Autodesk Inventor part; units mm, degrees
ref_plane "YZ Plane" through (0, 0, 0) normal (1, 0, 0) x (0, 1, 0)
ref_plane "XZ Plane" through (0, 0, 0) normal (0, 1, 0) x (-1, 0, 0)
ref_plane "XY Plane" through (0, 0, 0) normal (0, 0, 1) x (1, 0, 0)
sketch "Sketch1" plane through (0, 0, 0) normal (0, 0, 1) x (1, 0, 0)
  line L0 (-17, 28) -> (0, 28)
  line L1 (0, 28) -> (0, 0)
  line L2 (0, 0) -> (-17, 0)
  line L3 (-17, 0) -> (-17, 28)
  dimension "d0" = 17
  dimension "d1" = 28
extrude "Extrusion1" add sketch "Sketch1" along normal blind 1
sketch "Sketch2" plane through (0, 0, 1) normal (0, 0, 1) x (1, 0, 0)
  line L0 (-17, 28) -> (-17, 0)
  line L1 (0, 28) -> (-17, 28)
  line L2 (0, 0) -> (0, 28)
  line L3 (-17, 0) -> (0, 0)
  circle A0 centre (-12.5, 26) radius 1.35
  circle A1 centre (-4.5, 5) radius 1.35
  dimension "d4" = 2.7
  dimension "d5" = 2.7
  dimension "d6" = 4.5
  dimension "d7" = 4.5
  dimension "d8" = 2
  dimension "d9" = 5
extrude "Extrusion2" cut sketch "Sketch2" against normal through all contours A0 | A1
sketch "Sketch3" plane through (0, 0, 1) normal (0, 0, 1) x (1, 0, 0)
  circle A0 centre (-12.5, 26) radius 1.35
  circle A1 centre (-4.5, 5) radius 1.35
  line L0 (0, 28) -> (-17, 28)
  line L1 (-17, 28) -> (-17, 0)
  line L2 (-17, 0) -> (0, 0)
  line L3 (0, 0) -> (0, 28)
  circle A2 centre (-8.5, 12.047) radius 6.5
  dimension "d12" = 13
  dimension "d13" = 12.047
extrude "Extrusion3" add sketch "Sketch3" along normal blind 30 contours A2
sketch "Sketch4" plane through (-8.5, 12.047, 31) normal (0, 0, 1) x (1, 0, 0)
  circle A0 centre (0, 0) radius 6.5
  circle A1 centre (0, 0) radius 3.25
  point P0 (8.5, -12.047)
  dimension "d16" = 6.5
sketch "Sketch5" plane through (0, 0, 0) normal (0, 0, -1) x (-1, 0, 0)
  circle A0 centre (8.5, 12.047) radius 6.5
  circle A1 centre (8.5, 12.047) radius 5
  point P0 (0, 0)
  dimension "d17" = 10
loft "Loft1" cut profiles "Sketch5", "Sketch4" contours A1 / A1
sketch "Sketch6" plane through (-8.5, 12.047, 31) normal (0, 0, 1) x (1, 0, 0)
  circle A0 centre (0, 0) radius 3.25
  circle A1 centre (0, 0) radius 4.75
  point P0 (8.5, -12.047)
  dimension "d26" = 9.5
extrude "Extrusion6" add sketch "Sketch6" along normal blind 3
sketch "Sketch7" plane through (-8.5, 12.047, 34) normal (0, 0, 1) x (1, 0, 0)
  circle A0 centre (0, 0) radius 3.25
  circle A1 centre (0, 0) radius 4.75
  line L0 (2, 0) -> (-2, 0)
  line L1 (-2, 0) -> (-2, 6)
  line L2 (-2, 6) -> (2, 6)
  line L3 (2, 6) -> (2, 0)
  point P0 (8.5, -12.047)
  dimension "d29" = 4
  dimension "d30" = 2
extrude "Extrusion7" cut sketch "Sketch7" against normal up to surface (3 mm away) contours L3 L0 L1 A0 | A0 L1 A1 L3 | A1 L1 L2 L3 picked at (0, 1.0833) picked at (0.3414, 4.2128)
properties part number "TORRE0.2"
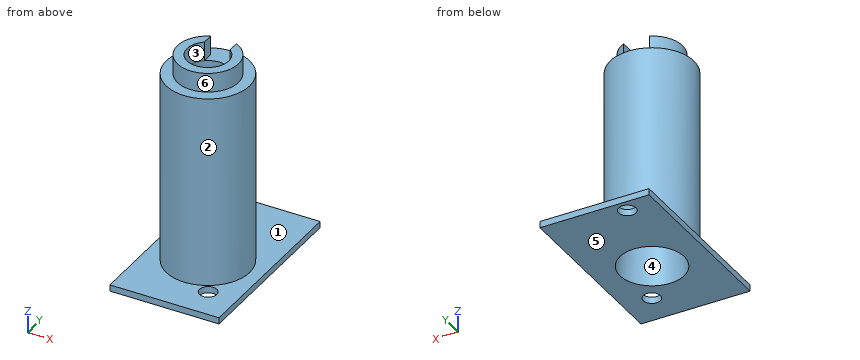
Build history of the part. All positions in model axes, mm. Face numbers are marked on the shaded views. A direction names the side the tool comes from. Give positions to 0.01 mm unless a question says otherwise; leave off trailing zeros. Write each loop counter-clockwise with the first axis right and the second up, starting at its lowest first coordinate (ties: lowest second). Pieces come first, ordered by that corner, then holes. Notation, with made-up numbers: (61.5, 40.25) - (72.5, 40.25) arc R21 ccw to (72.5, 60.25) - close; hole circle Ø8 at (86.25, 73.25). An arc over 180 degrees is marked (long way). Use one line per item in the form item = value. Start each with the question number.
1. Band-saw the part on B-B on x = -8.5. Write the cut outline in (y, z).
2. Band-saw the part on A-A on y = 26. Write the cut outline in (x, z).
3. Drop flat-ended pins along their axis: pin 1 Ø4 at (x, y) = (-5, 23.5) entering from +Z; pin 2 Ø6 at (y, z) = (12.5, 29.5) entering from +X; pin 3 Ø3 at (x, y) = (-10.5, 16) entering from -Z; pin 4 Ø3 at (x, y) = (-2.5, 7) entering from +Z. Give the stop position or say it passes through.
4. Band-saw the part on C-C on z = 12. Write the cut outline in (x, y).
5. Band-saw the part on D-D on y = 20. Write the cut outline in (x, z).
6. Two-plate mould, pull along X, no slides. Class the marked faces 1, 2, 3 and 4: released by +X, released by -X, zero draft, split by the parting line, or undercut.
7. 3-axis set-ups, long thin cutter, end or side, ignore diameter. For the marked faces 5 and 6: which of +Z, -Z, +X, -X, +Y, -Y reach the whole face in a straight line?
8. Probe line 1 (Y direction, x = -12.5, z = 0.3); line 2 (Z direction, x = -3, y = 6.5); line 3 (Y direction, x = -4.5, z = 0.45). List the from-to ranges inside material, lowest first. Write a range as [from, to].
Conclusion:
q1.outline = (0, 0) - (7.05, 0) - (8.8, 31) - (8.8, 34) - (7.3, 34) - (7.3, 31) - (5.55, 31) - (5.55, 1) - (0, 1) - close; (15.3, 31) - (17.05, 0) - (28, 0) - (28, 1) - (18.55, 1) - (18.55, 31) - close
q2.outline = (-17, 0) - (-13.85, 0) - (-13.85, 1) - (-17, 1) - close; (-11.15, 0) - (0, 0) - (0, 1) - (-11.15, 1) - close
q3.pin_1 = 1
q3.pin_2 = -2
q3.pin_3 = 0
q3.pin_4 = 31
q4.outline = circle Ø13 at (-8.5, 12.05); hole circle Ø8.65 at (-8.5, 12.05)
q5.outline = (-17, 0) - (0, 0) - (0, 1) - (-17, 1) - close
q6.face_1 = zero draft
q6.face_2 = split by the parting line
q6.face_3 = undercut
q6.face_4 = undercut
q7.face_5 = -Z, +X, -X, +Y, -Y
q7.face_6 = +Z
q8.line_1 = [0, 9.08], [15.02, 24.65], [27.35, 28]
q8.line_2 = [0, 1]
q8.line_3 = [0, 3.65], [6.35, 9.09], [15, 28]
